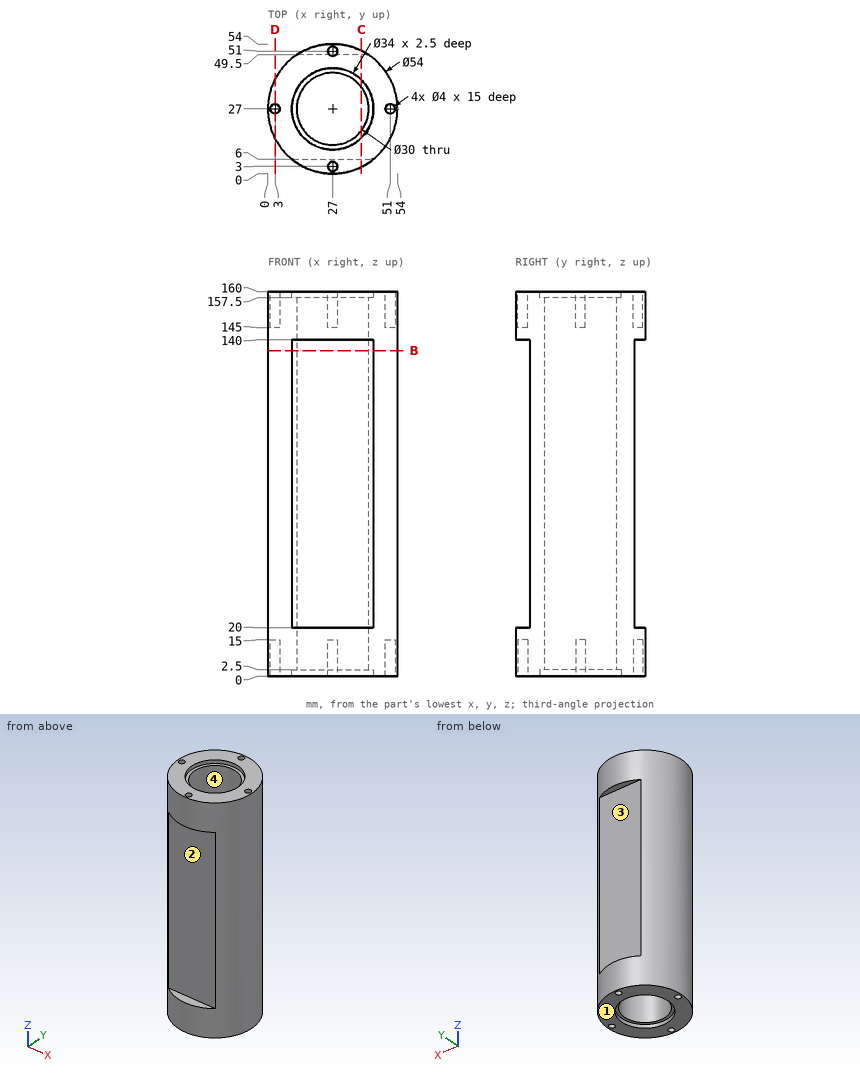
Input: dimensioned drawing with shaded views. Units: mm. Origin: part minimum x, y, z. Round coordinates to 2 decimals unless told otherwise and drop trailing zeros. Loops run counter-clockwise (first coordinate to the right, second up) from the corner with the lowest first, then second, coordinate; pieces in that order, holes last. Notation, with made-up numbers: (25, 6.5) -> (74, 6.5) arc R15 cw to (74, 24.5) -> close; hole circle Ø11 at (83, 9). An arc over 180 degrees is marked (long way). Answer as a JSON object with one key per item and string values. Group by question number.
Q1. Section query B-B (z = 135.5). Output: boundary loops of the cut face in (x, y).
Q2. Section query C-C (x = 39). Output: boundary loops of the cut face in (y, z), plus the area to 3 significant figures.
Q3. Section query D-D (x = 3). Output: boundary loops of the cut face in (y, z).
Q4. Contact query for flat-ended pins moving along their axis: P1, Ø2, axis at x = 18.5, z = 18.5, coming from the -Y side; P2, Ø1.5, axis at x = 38, z = 131, coming from the +Y side; P3, Ø1.2, axis at x = 27, y = 2, coming from the +Z side; P4, Ø3, axis at x = 31.5, y = 3, coming from the -Z side. Output: stop coordinate, or through.
Q5. Ray query, line 1 (Y direction, x = 27, z = 159.35); line 2 (Y direction, x = 27, z = 151.25); line 3 (Y direction, x = 27, z = 45). Return the intervals inside material, ascending. Write a range as from..to.
Q6. Mould query, pull axis Y, two halves, no side actions, for the marked faces 1, 2, 3 and 4. Classes: pulls with the +Y half, pulls with the -Y half, needs draft (parallel to the pull), parting line crosses it, or undercut.
Completed:
{
 "1": {"outline": "(10.03, 6) -> (43.97, 6) arc R27 ccw to (41.92, 49.5) -> (12.08, 49.5) arc R27 ccw to start; hole circle Ø30 at (27, 27)"},
 "2": {"outline": "(2.81, 0) -> (14.96, 0) -> (14.96, 2.5) -> (18, 2.5) -> (18, 157.5) -> (14.96, 157.5) -> (14.96, 160) -> (2.81, 160) -> (2.81, 140) -> (6, 140) -> (6, 20) -> (2.81, 20) -> close; (36, 2.5) -> (39.04, 2.5) -> (39.04, 0) -> (51.19, 0) -> (51.19, 20) -> (49.5, 20) -> (49.5, 140) -> (51.19, 140) -> (51.19, 160) -> (39.04, 160) -> (39.04, 157.5) -> (36, 157.5) -> close", "area": "4,240 mm²"},
 "3": {"outline": "(14.63, 0) -> (25, 0) -> (25, 15) -> (29, 15) -> (29, 0) -> (39.37, 0) -> (39.37, 160) -> (29, 160) -> (29, 145) -> (25, 145) -> (25, 160) -> (14.63, 160) -> close"},
 "4": {"P1": "y = 1.06", "P2": "y = 49.5", "P3": "z = 145", "P4": "z = 0"},
 "5": {"line 1": "0..1, 5..10, 44..49, 53..54", "line 2": "0..1, 5..12, 42..49, 53..54", "line 3": "6..12, 42..49.5"},
 "6": {"face 1": "needs draft", "face 2": "pulls with the -Y half", "face 3": "pulls with the +Y half", "face 4": "undercut"}
}
